Can you work these out from the model? Positions are in its coordinate system, mm. Face numbers are marked on the shaded views. A direction names the side the tool comes from. Coordinates: 2 decimals unless noted, no trailing zeros. Order: outer loops, then holes, each group sorted by start corner. A loop starts at its lowest first (then second) coordinate and runs counter-clockwise, first axis right, second up. Notation, with made-up numbers: (82.5, 81.5) - (105.5, 81.5) arc R21 cw to (105.5, 119.5) - close; hole circle Ø10 at (11, 19.25). An arc over 180 degrees is marked (long way). Use a Markdown table: item, result. Add a question column.
(1) I want a section at D-D (y = 5.75). List the corners of the cut face in (x, z) for me.
(2) For pin 1 Ø1 at (y, z) = (8, 0.5) entering from +X; pin 2 Ø1.5 at (y, z) = (9.5, 2) entering from -X, each with a flat end and sliding along its axis, tell me the tip position at first contact or that it passes through.
(3) I want a section at A-A (x = 0). List the corners of the cut face in (y, z) for me, and give its area (3 significant figures).
(4) If I drill on L1, parallel to X at y = 9.25, z = 0; L2, parallel to X at y = 5.75, z = 0, over which ranges is the centre line in solid material (lowest first)? Write a range as [from, to].
(5) We'd pull the mould along X, two halves only. Please class the marked faces 1, 2 and 3: pulls with the +X half, pulls with the -X half, needs draft (parallel to the pull), parting line crosses it, or undercut.
(6) I want a section at C-C (z = 2.75). List the corners of the cut face in (x, y) for me, and give its area (3 significant figures).
(7) On a 3-axis mill with a long thin cutter (end or side, diameter ignored), from which of +Z, -Z, +X, -X, +Y, -Y can I reach the whole of each face in a straight line? I mean the marked faces 4 and 5. Say none if no direction works.
(8) I want a section at B-B (z = 0). List the corners of the cut face in (x, y) for me, and give its area (3 significant figures).
Autodesk Inventor part; units mm, degrees
ref_plane "YZ Plane" through (0, 0, 0) normal (1, 0, 0) x (0, 1, 0)
ref_plane "XZ Plane" through (0, 0, 0) normal (0, 1, 0) x (-1, 0, 0)
ref_plane "XY Plane" through (0, 0, 0) normal (0, 0, 1) x (1, 0, 0)
sketch "Boceto1" plane through (0, 0, 0) normal (0, 1, 0) x (-1, 0, 0)
  circle A0 centre (0, 0) radius 3.1
  dimension "d0" = 6.2
extrude "Extrusión1" add sketch "Boceto1" along normal blind 11.5
sketch "Boceto2" plane through (0, 11.5, 0) normal (0, 1, 0) x (1, 0, 0)
  circle A0 centre (0, 0) radius 3.1
  circle A1 centre (0, 0) radius 2
  dimension "d3" = 4
extrude "Extrusión2" cut sketch "Boceto2" against normal blind 15.75 contours A1
sketch "Boceto3" plane through (0, 11.5, 0) normal (0, 1, 0) x (1, 0, 0)
  circle A0 centre (0, 0) radius 3
  circle A1 centre (0, 0) radius 4.9518
  dimension "d6" = 6
extrude "Extrusión3" cut sketch "Boceto3" against normal blind 5
equation "\"Radio_pliegue\" = Grosor"
equation "\"Anchura_desahogo_plegado\" = Grosor"
equation "\"Profundidad_desahogo_plegado\" = 0.5 * Grosor"
equation "\"Tamaño_destalonado\" = 4 * Grosor"
equation "\"Remanente_mínimo\" = 2 * Grosor"
equation "\"Radiodetransición\" = Radio_pliegue"
equation "\"Tamaño_de_radio_de_Jacobi\" = Radio_pliegue"
equation "\"TamañoSeparación\" = Grosor"
properties part number "Soporte de llanta"
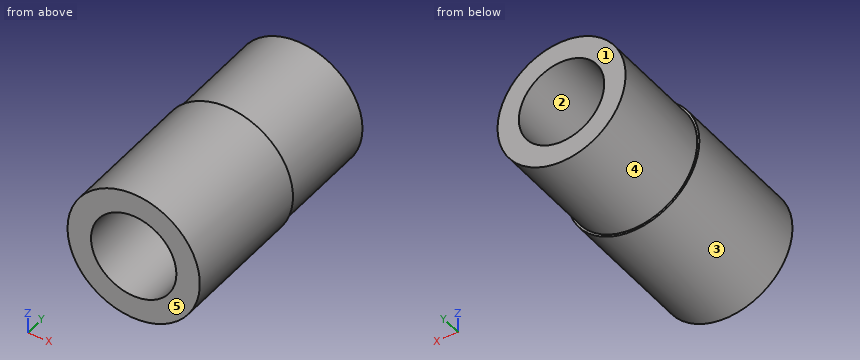
Answers follow:
| question | item | result |
|---|---|---|
| 1 | outline | circle Ø6.2 at (0, 0); hole circle Ø4 at (0, 0) |
| 2 | pin 1 | stops at x = 3 |
| 2 | pin 2 | stops at x = -2.73 |
| 3 | outline | (0, -3.1) - (6.5, -3.1) - (6.5, -3) - (11.5, -3) - (11.5, -2) - (0, -2) - close; (0, 2) - (11.5, 2) - (11.5, 3) - (6.5, 3) - (6.5, 3.1) - (0, 3.1) - close |
| 3 | area | 24.3 mm² |
| 4 | L1 | x = [-3, -2], [2, 3] |
| 4 | L2 | x = [-3.1, -2], [2, 3.1] |
| 5 | face 1 | needs draft |
| 5 | face 2 | undercut |
| 5 | face 3 | parting line crosses it |
| 6 | outline | (-1.43, 0) - (1.43, 0) - (1.43, 6.5) - (1.2, 6.5) - (1.2, 11.5) - (-1.2, 11.5) - (-1.2, 6.5) - (-1.43, 6.5) - close |
| 6 | area | 30.6 mm² |
| 7 | face 4 | +Y |
| 7 | face 5 | +Z, -Z, +X, -X, -Y |
| 8 | outline | (-3.1, 0) - (-2, 0) - (-2, 11.5) - (-3, 11.5) - (-3, 6.5) - (-3.1, 6.5) - close; (2, 0) - (3.1, 0) - (3.1, 6.5) - (3, 6.5) - (3, 11.5) - (2, 11.5) - close |
| 8 | area | 24.3 mm² |
